Input: part model. Units: mm. Frame: model coordinates. Face numbers are marked on the shaded views. A direction names the side the tool comes from. Coordinates: 2 decimals unless noted, no trailing zeros. Loops run counter-clockwise (first coordinate to the right, second up) from the corner with the lowest first, then second, coordinate; pieces in that order, holes last. Notation, with made-up numbers: (-38.5, 57.25) - (13.5, 57.25) arc R14 cw to (13.5, 73.25) - close; hole circle Ø1 at (65, -8.5). An arc over 180 degrees is marked (long way). Answer as CSV lines item,"result". Start each with the question number.
```python
from build123d import *

# Parameters (mm, degrees)
SKETCH1_W           = 25
SKETCH1_H           = 21
BOSS_EXTRUDE1_DEPTH = 15
SKETCH2_W           = 15
SKETCH2_H           = 3.4
CUT_EXTRUDE1_DEPTH  = 22.6
CUT_EXTRUDE2_DEPTH  = 5
FILLET1_R           = 1


with BuildPart() as part:
    # Sketch1 → Boss-Extrude1 (new body)
    with BuildSketch(Plane(origin=(0, 0, 0), x_dir=(1, 0, 0), z_dir=(0, 1, 0))):
        Rectangle(SKETCH1_W, SKETCH1_H)
    extrude(amount=BOSS_EXTRUDE1_DEPTH)

    # Sketch2 → Cut-Extrude1 (cut)
    with BuildSketch(Plane.ZY.offset(12.5)):
        with Locations((-3, 3.7)):
            Rectangle(SKETCH2_W, SKETCH2_H)
    extrude(amount=-CUT_EXTRUDE1_DEPTH, mode=Mode.SUBTRACT)

    # Sketch3 → Cut-Extrude2 (cut)
    with BuildSketch(Plane(origin=(0, 15, 0), x_dir=(1, 0, 0), z_dir=(0, 1, 0))):
        Polygon((-4.85, -0.925), (-4.85, -8.575), (-7.5, -8.575), (-7.5, -6.325), (-12.5, -6.325), (-12.5, -3.175), (-7.5, -3.175), (-7.5, -0.925), align=None)
        Polygon((-3.575, 10.5), (-0.425, 10.5), (-0.425, 5.5), (1.825, 5.5), (1.825, 2.85), (-5.825, 2.85), (-5.825, 5.5), (-3.575, 5.5), align=None)
    extrude(amount=-CUT_EXTRUDE2_DEPTH, mode=Mode.SUBTRACT)

    # Fillet1
    fillet1_edges = [part.edges().sort_by_distance(p)[0] for p in [
        (-7.5, 12.5, 6.325),
        (-12.5, 12.5, 6.325),
        (-12.5, 12.5, 3.175),
        (-7.5, 12.5, 3.175),
        (-6.175, 15, 0.925),
        (-7.5, 15, 2.05),
        (-10, 15, 3.175),
        (-10, 15, 6.325),
        (-7.5, 15, 7.45),
        (-6.175, 15, 8.575),
        (-4.85, 15, 4.75),
        (-3.575, 12.5, -5.5),
        (-0.425, 12.5, -5.5),
        (-3.575, 15, -8),
        (-4.7, 15, -5.5),
        (-5.825, 15, -4.175),
        (-2, 15, -2.85),
        (1.825, 15, -4.175),
        (0.7, 15, -5.5),
        (-0.425, 15, -8),
    ]]
    fillet(fillet1_edges, radius=FILLET1_R)


solid = part.part
```
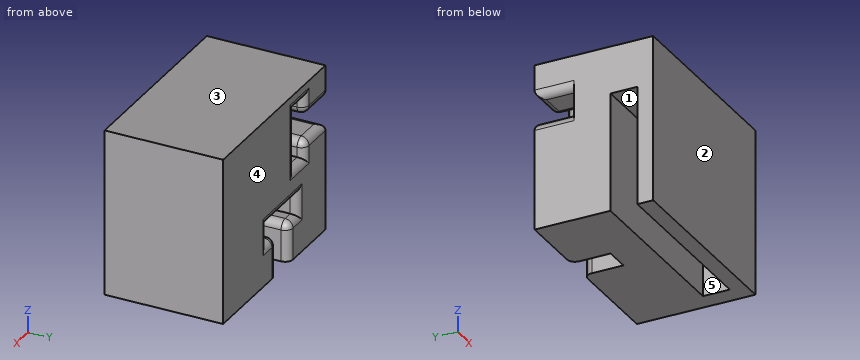
Item 1: Section query B-B, the plane x = -10. Output: boundary loops of the cut face in (y, z) (3 decimals), and give its area (3 significant figures).
Item 2: Section query C-C, the plane y = 2.75. Output: boundary loops of the cut face in (x, z).
Item 3: Draft query along Y for the marked faces 3, 4 and 5. Return one class per face: pulls with the +Y half, pulls with the -Y half, needs draft (parallel to the pull), parting line crosses it, or undercut.
Item 4: Section query A-A, the plane z = -3.25. Output: boundary loops of the cut face in (x, y) (3 decimals).
Item 5: Set-up query: the marked faces 1 and 2. Return all of +Z, -Z, +X, -X, +Y, -Y with unobstructed straight access to the full face (end or side cutting, diameter ignored); none if empty.
Item 6: Material intervals for probe 1 along Z at (x, y) = (-5, 11.25) (3 decimals); probe 2 along Y at (x, z) = (-5.5, -4.5); probe 3 along Y at (x, z) = (8, -0.5), sorted ascending.
Item 7: Section query D-D, the plane x = 7. Output: boundary loops of the cut face in (y, z).
Item 8: Contact query for flat-ended pins moving along their axis: P1, Ø1.7, axis at y = 3.5, z = -1, coming from the -X side; P2, Ø2.5, axis at x = -2, y = 4, coming from the -Z side. Output: stop coordinate, or through.
Response values:
1,outline,"(0, -10.5) - (2, -10.5) - (2, 4.5) - (5.4, 4.5) - (5.4, -10.5) - (15, -10.5) - (15, 2.175) arc R1 ccw to (14, 3.175) - (10, 3.175) - (10, 6.325) - (14, 6.325) arc R1 ccw to (15, 7.325) - (15, 10.5) - (0, 10.5) - close"
1,area,"248 mm²"
2,outline,"(-12.5, 4.5) - (10.1, 4.5) - (10.1, -10.5) - (12.5, -10.5) - (12.5, 10.5) - (-12.5, 10.5) - close"
3,face 3,"needs draft"
3,face 4,"pulls with the +Y half"
3,face 5,"undercut"
4,outline,"(-12.5, 0) - (12.5, 0) - (12.5, 15) - (2.825, 15) arc R1 ccw to (1.825, 14) - (1.825, 10) - (-5.825, 10) - (-5.825, 14) arc R1 ccw to (-6.825, 15) - (-12.5, 15) - (-12.5, 5.4) - (10.1, 5.4) - (10.1, 2) - (-12.5, 2) - close"
5,face 1,"-Z, -X"
5,face 2,"+Z, -Z, +X, -X, -Y"
6,probe 1,"z = -10.5 to -5.5, -2.85 to 0.925, 8.575 to 10.5"
6,probe 2,"y = 0 to 2, 5.4 to 10"
6,probe 3,"y = 0 to 2, 5.4 to 15"
7,outline,"(0, -10.5) - (2, -10.5) - (2, 4.5) - (5.4, 4.5) - (5.4, -10.5) - (15, -10.5) - (15, 10.5) - (0, 10.5) - close"
8,P1,"stops at x = 10.1"
8,P2,"stops at z = 4.5"
